from build123d import *

# Parameters (mm, degrees)
F0_W           = 1638.3
F0_H           = 723.9
F1_DEPTH       = 19.05
F2_W           = 1638.3
F2_H           = 723.9
F3_DEPTH       = 139.7
F5_W           = 1562.1
F5_H           = 647.7
F6_DEPTH       = 139.7
F4_W           = 88.9
F4_H           = 88.9
F7_DEPTH       = 139.7
F7_DEPTH_BACK  = 622.3
F8_W           = 38.1
F8_H           = 139.7
F9_DEPTH       = 647.7
F10_W          = 38.1
F10_H          = 139.7
F11_DEPTH      = 647.7
F12_SIZE       = 19.05
F13_R          = 9.525
F14_DEPTH      = 6.35
F14_DEPTH_BACK = 76.2
F15_W          = 139.7
F15_H          = 38.1
F16_DEPTH      = 1308.1
F17_W          = 38.1
F17_H          = 38.1
F18_DEPTH      = 1384.3
F19_W          = 38.1
F19_H          = 38.1
F20_DEPTH      = 469.9
F21_W          = 38.1
F21_H          = 40.64
F22_DEPTH      = 520.7
F23_W          = 38.1
F23_H          = 38.1
F24_DEPTH      = 1384.3
F25_R          = 9.525
F26_DEPTH      = 6.35
F26_DEPTH_BACK = 76.2
F27_R          = 9.525
F28_DEPTH      = 6.35
F28_DEPTH_BACK = 76.2
F29_R          = 9.525
F30_DEPTH      = 6.35
F30_DEPTH_BACK = 76.2
F31_R          = 9.525
F32_DEPTH      = 6.35
F32_DEPTH_BACK = 76.2


with BuildPart() as f1:
    # F0 (on Front) → F1 (new body)
    with BuildSketch(Plane.XZ):
        Rectangle(F0_W, F0_H)
    extrude(amount=F1_DEPTH)

    # F2 (on face) → F3 (join)
    with BuildSketch(Plane(origin=(0, 0, 0), x_dir=(-1, 0, 0), z_dir=(0, 1, 0))):
        Rectangle(F2_W, F2_H)
    extrude(amount=F3_DEPTH)

    # F5 (on face) → F6 (cut)
    with BuildSketch(Plane(origin=(0, 139.7, 0), x_dir=(-1, 0, 0), z_dir=(0, 1, 0))):
        Rectangle(F5_W, F5_H)
    extrude(amount=-F6_DEPTH, mode=Mode.SUBTRACT)

    # F4 (on face) → F7 (join, two sides)
    with BuildSketch(Plane(origin=(0, 139.7, 0), x_dir=(-1, 0, 0), z_dir=(0, 1, 0))) as f7_sk:
        with Locations((-736.6, 279.4)):
            Rectangle(F4_W, F4_H)
        with Locations((736.6, 279.4)):
            Rectangle(F4_W, F4_H)
        with Locations((736.6, -279.4)):
            Rectangle(F4_W, F4_H)
        with Locations((-736.6, -279.4)):
            Rectangle(F4_W, F4_H)
    extrude(amount=-F7_DEPTH)
    extrude(f7_sk.sketch, amount=F7_DEPTH_BACK)

    # F8 (on face) → F9 (join)
    with BuildSketch(Plane.XY.offset(323.85)):
        with Locations((-673.1, 488.95)):
            Rectangle(F8_W, F8_H)
    extrude(amount=-F9_DEPTH)

    # F10 (on face) → F11 (join)
    with BuildSketch(Plane.XY.offset(323.85)):
        with Locations((673.1, 488.95)):
            Rectangle(F10_W, F10_H)
    extrude(amount=-F11_DEPTH)

    # F12
    f12_edges = [f1.edges().sort_by_distance(p)[0] for p in [
        (736.6, 762, -323.85),
        (781.05, 762, -279.4),
        (736.6, 762, -234.95),
        (692.15, 762, -279.4),
        (736.6, 762, 323.85),
        (692.15, 762, 279.4),
        (781.05, 762, 279.4),
        (736.6, 762, 234.95),
        (-736.6, 762, 323.85),
        (-736.6, 762, 234.95),
        (-692.15, 762, 279.4),
        (-781.05, 762, 279.4),
        (-736.6, 762, -234.95),
        (-781.05, 762, -279.4),
        (-736.6, 762, -323.85),
        (-692.15, 762, -279.4),
    ]]
    chamfer(f12_edges, length=F12_SIZE)

    # F13 (on face) → F14 (join, two sides)
    with BuildSketch(Plane.XY.offset(361.95)) as f14_sk:
        with Locations((-755.65, 101.6)):
            Circle(F13_R)
        with Locations((-717.55, 63.5)):
            Circle(F13_R)
    extrude(amount=F14_DEPTH)
    extrude(f14_sk.sketch, amount=-F14_DEPTH_BACK)

    # F15 (on face) → F16 (join)
    with BuildSketch(Plane(origin=(654.05, 0, 0), x_dir=(0, -1, 0), z_dir=(-1, 0, 0))):
        with Locations((-488.95, 0)):
            Rectangle(F15_W, F15_H)
    extrude(amount=F16_DEPTH)

    # F17 (on face) → F18 (join)
    with BuildSketch(Plane.YZ.offset(-692.15)):
        with Locations((19.05, -304.8)):
            Rectangle(F17_W, F17_H)
    extrude(amount=F18_DEPTH)

    # F19 (on face) → F20 (join)
    with BuildSketch(Plane.XY.offset(-234.95)):
        with Locations((762, 19.05)):
            Rectangle(F19_W, F19_H)
    extrude(amount=F20_DEPTH)

    # F21 (on face) → F22 (join)
    with BuildSketch(Plane.XY.offset(-234.95)):
        with Locations((-762, 20.32)):
            Rectangle(F21_W, F21_H)
    extrude(amount=F22_DEPTH)

    # F23 (on face) → F24 (join)
    with BuildSketch(Plane.YZ.offset(-692.15)):
        with Locations((19.05, 304.8)):
            Rectangle(F23_W, F23_H)
    extrude(amount=F24_DEPTH)

    # F25 (on face) → F26 (join, two sides)
    with BuildSketch(Plane.XY.offset(361.95)) as f26_sk:
        with Locations((717.55, 101.6)):
            Circle(F25_R)
        with Locations((755.65, 63.5)):
            Circle(F25_R)
    extrude(amount=F26_DEPTH)
    extrude(f26_sk.sketch, amount=-F26_DEPTH_BACK)

    # F27 (on face) → F28 (join, two sides)
    with BuildSketch(Plane(origin=(-819.15, 0, 0), x_dir=(0, -1, 0), z_dir=(-1, 0, 0))) as f28_sk:
        with Locations((-101.6, 260.35)):
            Circle(F27_R)
        with Locations((-63.5, 298.45)):
            Circle(F27_R)
        with Locations((-101.6, -298.45)):
            Circle(F27_R)
        with Locations((-63.5, -260.35)):
            Circle(F27_R)
    extrude(amount=F28_DEPTH)
    extrude(f28_sk.sketch, amount=-F28_DEPTH_BACK)

    # F29 (on face) → F30 (join, two sides)
    with BuildSketch(Plane.YZ.offset(819.15)) as f30_sk:
        with Locations((101.6, 298.45)):
            Circle(F29_R)
        with Locations((101.6, -260.35)):
            Circle(F29_R)
        with Locations((63.5, 260.35)):
            Circle(F29_R)
        with Locations((63.5, -298.45)):
            Circle(F29_R)
    extrude(amount=F30_DEPTH)
    extrude(f30_sk.sketch, amount=-F30_DEPTH_BACK)

    # F31 (on face) → F32 (join, two sides)
    with BuildSketch(Plane(origin=(0, 0, -361.95), x_dir=(1, 0, 0), z_dir=(0, 0, -1))) as f32_sk:
        with Locations((-755.65, -63.5)):
            Circle(F31_R)
        with Locations((-717.55, -101.6)):
            Circle(F31_R)
        with Locations((717.55, -63.5)):
            Circle(F31_R)
        with Locations((755.65, -101.6)):
            Circle(F31_R)
    extrude(amount=F32_DEPTH)
    extrude(f32_sk.sketch, amount=-F32_DEPTH_BACK)


solid = f1.part
Model file for the job. Use its own axes, mm. A direction names the side the tool comes from. Give positions to 0.01 mm unless a question says otherwise; leave off trailing zeros. Order: outer loops, then holes, each group sorted by start corner. A loop starts at its lowest first (then second) coordinate and runs counter-clockwise, first axis right, second up. Notation, with made-up numbers: M 21,89.25 L 79,89.25 A19 cw 79,126.25 Z; hole C -6.75,79 d10. An arc over 180 degrees is marked long. Write item = value, one per line.
Q1. Drill centre lines: line 1 (Z direction, x = 230, y = 98.5); line 2 (X direction, y = 270, z = 272.5); line 3 (Y direction, x = 542, z = -11). Where is each one in solid material? Low to high. Write a range as [from, to].
Derived:
line_1 = [-361.95, -323.85], [323.85, 361.95]
line_2 = [-781.05, -692.15], [692.15, 781.05]
line_3 = [-19.05, 0], [419.1, 558.8]
Q2. Two-plate mould, pull along X, no slides. Class faces 1 (the flat face through (-733, 446, 323.85)), 2 (the flat face through (-654.05, 488, 174)), 3 (the flat face through (819.15, 59, -5)): pulls with the +X half, pulls with the -X half, needs draft (parallel to the pull), parting line crosses it, or undercut.
Derived:
face_1 = needs draft
face_2 = undercut
face_3 = pulls with the +X half
Q3. Flat gauge pins, fed straight in: pin 1 (1 mm diameter, centred on x = -228, y = 423, fed in from -Z); pin 2 (1.5 mm diameter, centred on y = 469, z = 133, fed in from -X); pin 3 (10 mm diameter, centred on x = -284, z = 167.5, fed in from +Y). Where does each tip first touch, or does it go through?
Derived:
pin_1 = -19.05
pin_2 = -692.15
pin_3 = 0
Q4. Cut at A-A, the plane y = 628.5. List the corners of the cut face in (x, z), then the cut area to 3 significant figures.
Derived:
outline = M -781.05,-323.85 L -692.15,-323.85 L -692.15,-234.95 L -781.05,-234.95 Z; M -781.05,234.95 L -692.15,234.95 L -692.15,323.85 L -781.05,323.85 Z; M 692.15,-323.85 L 781.05,-323.85 L 781.05,-234.95 L 692.15,-234.95 Z; M 692.15,234.95 L 781.05,234.95 L 781.05,323.85 L 692.15,323.85 Z
area = 31,600 mm2
Q5. Cut at C-C, the plane z = 214. List the corners of the cut face in (x, y).
Derived:
outline = M -819.15,-19.05 L 819.15,-19.05 L 819.15,139.7 L 781.05,139.7 L 781.05,38.1 L 742.95,38.1 L 742.95,0 L -742.95,0 L -742.95,40.64 L -781.05,40.64 L -781.05,139.7 L -819.15,139.7 Z; M -692.15,419.1 L -654.05,419.1 L -654.05,558.8 L -692.15,558.8 Z; M 654.05,419.1 L 692.15,419.1 L 692.15,558.8 L 654.05,558.8 Z
Q6. Cut at B-B, the plane x = 318.5. List the corners of the cut face in (y, z), then the cut area to 3 significant figures.
Derived:
outline = M -19.05,-361.95 L 139.7,-361.95 L 139.7,-323.85 L 38.1,-323.85 L 38.1,-285.75 L 0,-285.75 L 0,285.75 L 38.1,285.75 L 38.1,323.85 L 139.7,323.85 L 139.7,361.95 L -19.05,361.95 Z; M 419.1,-19.05 L 558.8,-19.05 L 558.8,19.05 L 419.1,19.05 Z
area = 32,700 mm2
Q7. Tool access for faces 4 (the flat face through (-692.15, 652, -280)), 5 (the flat face through (692.15, 207, -280)), 6 (the flat face through (-736, 377, 234.95)): list every direction of +Z, -Z, +X, -X, +Y, -Y with a clear straight run to the whole face (end or side of a thin tool).
Derived:
face_4 = +Z, -Z, +Y
face_5 = none
face_6 = +Y
